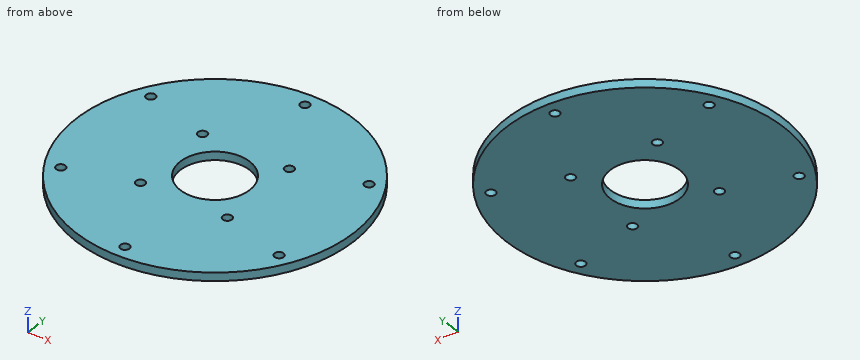
```python
from build123d import *

# Parameters (mm, degrees)
SKETCH_1_R      = 50
SKETCH_1_R_2    = 1.65
SKETCH_1_R_3    = 12.5
EXTRUDE_1_DEPTH = 3


with BuildPart() as part:
    # 草图1 → 凸台-拉伸1 (new body)
    with BuildSketch(Plane.XY):
        Circle(SKETCH_1_R)
        with Locations((-15.5, 15.5)):
            Circle(SKETCH_1_R_2, mode=Mode.SUBTRACT)
        with Locations((15.5, 15.5)):
            Circle(SKETCH_1_R_2, mode=Mode.SUBTRACT)
        with Locations((15.5, -15.5)):
            Circle(SKETCH_1_R_2, mode=Mode.SUBTRACT)
        with Locations((-15.5, -15.5)):
            Circle(SKETCH_1_R_2, mode=Mode.SUBTRACT)
        Circle(SKETCH_1_R_3, mode=Mode.SUBTRACT)
        with Locations((-38.97114317, 22.5)):
            Circle(SKETCH_1_R_2, mode=Mode.SUBTRACT)
        with Locations((0, 45)):
            Circle(SKETCH_1_R_2, mode=Mode.SUBTRACT)
        with Locations((38.97114317, 22.5)):
            Circle(SKETCH_1_R_2, mode=Mode.SUBTRACT)
        with Locations((38.97114317, -22.5)):
            Circle(SKETCH_1_R_2, mode=Mode.SUBTRACT)
        with Locations((0, -45)):
            Circle(SKETCH_1_R_2, mode=Mode.SUBTRACT)
        with Locations((-38.97114317, -22.5)):
            Circle(SKETCH_1_R_2, mode=Mode.SUBTRACT)
    extrude(amount=EXTRUDE_1_DEPTH)


solid = part.part
```
CAD build for the part. Positions are in the model's coordinates, mm. Coordinates: 2 decimals unless noted, no trailing zeros. Write each loop counter-clockwise with the first axis right and the second up, starting at its lowest first coordinate (ties: lowest second). Pieces come first, ordered by that corner, then holes.
(1) Drill centre lines: probe 1 along Y at (x, z) = (0, 2.4); probe 2 along Y at (x, z) = (-15.5, 1.55); probe 3 along Y at (x, z) = (39, 2.1). Where is each one in solid material? Low to high.
(2) Cut at B-B, the plane x = 0. List the corners of the cut face in (y, z).
(3) Cut at C-C, the plane z = 0.8. Count the separate pieces of the cut face and the enclosed holes in it, and give its area (3 significant figures).
(4) Cut at A-A, the plane y = 0. List the corners of the cut face in (x, z).
(5) Flat gauge pins, fed straight in: pin 1 (3 mm diameter, centred on x = 38.97, y = -22.5, fed in from -Z); pin 2 (4 mm diameter, centred on x = -38.97, y = 22.5, fed in from +Z); pin 3 (1 mm diameter, centred on y = 11, z = 2.5, fed in from -X). Where does each tip first touch, or does it go through?
(6) Cut at D-D, the plane y = -22.5. List the corners of the cut face in (x, z).
Geometry says:
1. probe 1: y = -50 to -46.65, -43.35 to -12.5, 12.5 to 43.35, 46.65 to 50
1. probe 2: y = -47.54 to -17.15, -13.85 to 13.85, 17.15 to 47.54
1. probe 3: y = -31.29 to -24.15, -20.85 to 20.85, 24.15 to 31.29
2. outline: (-50, 0) - (-46.65, 0) - (-46.65, 3) - (-50, 3) - close; (-43.35, 0) - (-12.5, 0) - (-12.5, 3) - (-43.35, 3) - close; (12.5, 0) - (43.35, 0) - (43.35, 3) - (12.5, 3) - close; (46.65, 0) - (50, 0) - (50, 3) - (46.65, 3) - close
3. separate pieces: 1
3. enclosed holes: 11
3. area: 7,280 mm2
4. outline: (-50, 0) - (-12.5, 0) - (-12.5, 3) - (-50, 3) - close; (12.5, 0) - (50, 0) - (50, 3) - (12.5, 3) - close
5. pin 1: passes through
5. pin 2: stops at z = 3
5. pin 3: stops at x = -48.89
6. outline: (-44.65, 0) - (-40.62, 0) - (-40.62, 3) - (-44.65, 3) - close; (-37.32, 0) - (37.32, 0) - (37.32, 3) - (-37.32, 3) - close; (40.62, 0) - (44.65, 0) - (44.65, 3) - (40.62, 3) - close
